Design review of the part built by this model. Coordinates are the model's own, in mm. A direction names the side the tool comes from. Coordinates: 2 decimals unless noted, no trailing zeros. Loops run counter-clockwise (first coordinate to the right, second up) from the corner with the lowest first, then second, coordinate; pieces in that order, holes last. Notation, with made-up numbers: (-30, 60.25) -> (29, 60.25) arc R32 cw to (29, 88.25) -> close; hole circle Ø10 at (43, 59). An arc over 180 degrees is marked (long way). Use a Markdown table: item, result. Add a question column.
Q1. Take a section at C-C on z = 13. Write out the cut boundary in (x, y).
Q2. Clearance check with flat-ended pins moving along their axes: pin 1 Ø0.6 at (x, y) = (-24.5, -0.5) entering from +Z; pin 2 Ø3 at (x, y) = (0, 0) entering from -Z; pin 3 Ø18 at (x, y) = (-2.5, 6.5) entering from +Z. State where each tip first meets the part, or that it passes through.
Q3. Take a section at D-D on y = 0. Write out the cut boundary in (x, z).
Q4. Take a section at B-B on y = 10.5. Write out the cut boundary in (x, z).
Q5. For probe 1 along Y at (x, z) = (-20.5, 15); probe 2 along X at (y, z) = (-8, 11.5); probe 3 along Y at (x, z) = (0, 0.55), list the stretches that pass through material, from the lowest coordinate up.
Q6. For faces 1 (the face through (-19, 18, 16.002)), 2 (the face through (24.13, 0, 8)), list the 3-axis set-ups (+Z, -Z, +X, -X, +Y, -Y) from which the entire face can be reached by the end or side of a thin tool; tool diameter is ignored.
Q7. Take a section at A-A on x = 0. Write out the cut boundary in (y, z), plus the area to 3 significant figures.
Q8. Draft analysis for pull direction Y (two halves, no side actions). For faces 3 (the face through (0, 18.542, 8)), 4 (the face through (24.892, 0, 8)), 5 (the face through (0.33, -2.52, 0.39)), 6 (the face through (0, -18.542, 8)), state which applies: pulls with the +Y half, pulls with the -Y half, needs draft (parallel to the pull), parting line crosses it, or undercut.
from build123d import *

# Parameters (mm, degrees)
F0_R      = 2.921
F1_DEPTH  = 16.002
F2_T      = -0.762
F3_D      = 6.858
F4_D      = 5.08
F5_W      = 8.128
F5_H      = 3.048
F6_DEPTH  = 25.4
F8_DEPTH  = 25.4
F10_DEPTH = 25.4


with BuildPart() as f1:
    # F0 (on Top) → F1 (new body)
    with BuildSketch(Plane.XY):
        Polygon((24.892, -18.542), (24.892, 18.542), (-24.892, 18.542), (-24.892, 0), (-24.892, -18.542), align=None)
        with BuildLine():
            ThreePointArc((-12.573, 0), (-16.383, -3.81), (-20.193, 0))
            ThreePointArc((-20.193, 0), (-16.383, 3.81), (-12.573, 0))
        make_face(mode=Mode.SUBTRACT)
        Circle(F0_R, mode=Mode.SUBTRACT)
        with BuildLine():
            ThreePointArc((-12.573, 0), (-16.383, 3.81), (-20.193, 0))
            ThreePointArc((-20.193, 0), (-16.383, -3.81), (-12.573, 0))
        make_face()
        Circle(F0_R)
    extrude(amount=F1_DEPTH)

    # F2
    f2_openings = [f1.faces().sort_by_distance(p)[0] for p in [
        (0, 0, 16.002),
    ]]
    offset(amount=F2_T, openings=f2_openings)

    # F3 (through all)
    with Locations(Plane(origin=(0, 0, 0), x_dir=(1, 0, 0), z_dir=(0, 0, -1))):
        with Locations((-16.383, 0)):
            Hole(F3_D / 2)

    # F4 (through all)
    with Locations(Plane(origin=(0, 0, 0), x_dir=(1, 0, 0), z_dir=(0, 0, -1))):
        with Locations((0, 0)):
            Hole(F4_D / 2)

    # F5 (on face) → F6 (cut)
    with BuildSketch(Plane.XZ.offset(18.542)):
        with Locations((15.494, 4.318)):
            Rectangle(F5_W, F5_H)
    extrude(amount=-F6_DEPTH, mode=Mode.SUBTRACT)

    # F7 (on face) → F8 (cut)
    with BuildSketch(Plane(origin=(0, 18.542, 0), x_dir=(-1, 0, 0), z_dir=(0, 1, 0))):
        Polygon((2.159, 10.16), (2.159, 16.002), (0, 16.002), (-2.159, 16.002), (-2.159, 10.16), align=None)
    extrude(amount=-F8_DEPTH, mode=Mode.SUBTRACT)

    # F9 (on face) → F10 (cut)
    with BuildSketch(Plane(origin=(-24.892, 0, 0), x_dir=(0, -1, 0), z_dir=(-1, 0, 0))):
        Polygon((2.159, 10.16), (2.159, 16.002), (0, 16.002), (-2.159, 16.002), (-2.159, 10.16), align=None)
    extrude(amount=-F10_DEPTH, mode=Mode.SUBTRACT)


solid = f1.part
Answer list:
| question | item | result |
|---|---|---|
| 1 | outline | (-24.89, -18.54) -> (24.89, -18.54) -> (24.89, 18.54) -> (2.16, 18.54) -> (2.16, 17.78) -> (24.13, 17.78) -> (24.13, -17.78) -> (-24.13, -17.78) -> (-24.13, -2.16) -> (-24.89, -2.16) -> close; (-24.89, 2.16) -> (-24.13, 2.16) -> (-24.13, 17.78) -> (-2.16, 17.78) -> (-2.16, 18.54) -> (-24.89, 18.54) -> close |
| 2 | pin 1 | z = 10.16 |
| 2 | pin 2 | through |
| 2 | pin 3 | z = 0.76 |
| 3 | outline | (-24.89, 0) -> (-19.81, 0) -> (-19.81, 0.76) -> (-24.13, 0.76) -> (-24.13, 10.16) -> (-24.89, 10.16) -> close; (-12.95, 0) -> (-2.54, 0) -> (-2.54, 0.76) -> (-12.95, 0.76) -> close; (2.54, 0) -> (24.89, 0) -> (24.89, 16) -> (24.13, 16) -> (24.13, 0.76) -> (2.54, 0.76) -> close |
| 4 | outline | (-24.89, 0) -> (24.89, 0) -> (24.89, 16) -> (24.13, 16) -> (24.13, 0.76) -> (-24.13, 0.76) -> (-24.13, 16) -> (-24.89, 16) -> close |
| 5 | probe 1 | -18.54 to -17.78, 17.78 to 18.54 |
| 5 | probe 2 | -24.89 to -24.13, 24.13 to 24.89 |
| 5 | probe 3 | -18.54 to -2.54, 2.54 to 18.54 |
| 6 | face 1 | +Z, +X, -X, +Y, -Y |
| 6 | face 2 | +Z |
| 7 | outline | (-18.54, 0) -> (-2.54, 0) -> (-2.54, 0.76) -> (-17.78, 0.76) -> (-17.78, 16) -> (-18.54, 16) -> close; (2.54, 0) -> (18.54, 0) -> (18.54, 10.16) -> (17.78, 10.16) -> (17.78, 0.76) -> (2.54, 0.76) -> close |
| 7 | area | 43.2 mm² |
| 8 | face 3 | pulls with the +Y half |
| 8 | face 4 | needs draft |
| 8 | face 5 | undercut |
| 8 | face 6 | pulls with the -Y half |
